Part model, mm, in its own coordinate system. A direction names the side the tool comes from. Give positions to 0.01 mm unless a question says otherwise; leave off trailing zeros. Order: outer loops, then holes, each group sorted by start corner. A loop starts at its lowest first (then second) coordinate and runs counter-clockwise, first axis right, second up. Notation, with made-up numbers: M 9.5,-15.5 L 66.5,-15.5 A16 cw 66.5,-11.5 Z; hole C 34,81.5 d1. An arc over 180 degrees is marked long. Return JSON: item names as keys, results as strings.
Autodesk Inventor part; units mm, degrees
ref_plane "YZ Plane" through (0, 0, 0) normal (1, 0, 0) x (0, 1, 0)
ref_plane "XZ Plane" through (0, 0, 0) normal (0, 1, 0) x (-1, 0, 0)
ref_plane "XY Plane" through (0, 0, 0) normal (0, 0, 1) x (1, 0, 0)
sketch "Boceto1" plane through (0, 0, 0) normal (0, 0, 1) x (1, 0, 0)
  line L0 (0, 0) -> (-1.5875, 0)
  line L1 (-1.4605, 11.9062) -> (0, 11.9062)
  line L2 (0, 11.9062) -> (0, 0)
  line L3 (-1.4605, 11.9062) -> (-1.5875, 11.7793)
  line L4 (-1.1906, 7.5375) -> (-1.1906, 6.7437)
  line L5 (-1.4605, 7.5375) -> (-1.1906, 7.5375)
  line L6 (-1.5875, 7.6645) -> (-1.5875, 11.7793)
  line L7 (-1.5875, 7.6645) -> (-1.4605, 7.5375)
  line L8 (0, 0) -> (-1.905, 0)
  line L9 (-2.3813, 6.7469) -> (-1.1906, 6.7469)
  line L10 (0, 6.7469) -> (0, 0)
  arc A0 (-2.3813, 2.4473) -> (-1.905, 0) centre (-1.905, 1.27) ccw
  line L11 (-2.3813, 0) -> (-2.3813, 0.0927)
  line L12 (-2.3813, 2.4473) -> (-2.3813, 6.7469)
  point P0 (-1.5875, 11.9062)
  point P1 (-1.5875, 7.5375)
  dimension "d0" = 1.5875
  dimension "d1" = 11.9062
  dimension "d2" = 0.127
  dimension "d3" = 0.127
  dimension "d5" = 0.7937
  dimension "d7" = 4.3688
  dimension "d8" = 0.127
  dimension "d9" = 0.127
  dimension "d10" = 2.3813
  dimension "d11" = 6.7469
  dimension "d12" = 2.54
  dimension "d13" = 1.27
  dimension "d14" = 1.905
revolve "Revolución1" add sketch "Boceto1" angle 360 about axis through (0, 11.9062, 0) along (0, -1, 0)
thread "Rosca1"
sketch "Boceto2" plane through (0, 0, 0) normal (0, -1, 0) x (1, 0, 0)
  line L0 (-0.3969, 3.9709) -> (0.3969, 3.9709)
  line L1 (0.3969, 3.9709) -> (0.3969, -4.5285)
  line L2 (0.3969, -4.5285) -> (-0.3969, -4.5285)
  line L3 (-0.3969, -4.5285) -> (-0.3969, 3.9709)
  point P0 (0, 0)
  dimension "d18" = 0.7937
  dimension "d19" = 0.3969
extrude "Extrusión1" cut sketch "Boceto2" against normal blind 0.7937
equation "\"d7\" = d4"
properties part number "Crank Screw" material "Acero inoxidable"
Q1. Band-saw the part on D-D (y = 10.25). Give the cut face in (x, z) (1 decimal), then the cut area to 3 significant figures.
Established:
{"outline": "C 0,0 d3.2", "area": "7.92 mm²"}
Q2. Probe line 1 along Z through (x, y) = (0, 3.25); line 2 along Y through (x, z) = (0.5, 1.25); line 3 along Y through (x, z) = (-1, 1.5). List the from-to ranges inside material, lowest first.
Established:
{"line 1": "z = -2.38 to 2.38", "line 2": "y = 0 to 6.75, 7.54 to 11.91", "line 3": "y = 0 to 6.75"}
Q3. Band-saw the part on C-C (y = 4.75). Give the cut face in (x, z), then the cut area to 3 significant figures.
Established:
{"outline": "C 0,0 d4.76", "area": "17.8 mm²"}
Q4. 3-axis set-ups, long thin cutter, end or side, ignore diameter. For faces 4 (the cylindrical face through (0.34, 9.75, -1.55)), 5 (the flat face through (1, 0, 0)), 6 (the flat face through (1, 6.747, -1)): which of +Z, -Z, +X, -X, +Y, -Y reach the whole face in a straight line?
Established:
{"face 4": "+Y", "face 5": "+Z, -Z, +X, -X, -Y", "face 6": "none"}
Q5. Pin check, flat tips, straight feed: pin 1 (3 mm diameter, centred on x = 2, z = 2.5, fed in from +Y); pin 2 (1 mm diameter, centred on x = -0.5, y = 8, fed in from -Z); pin 3 (1.5 mm diameter, centred on x = 2.5, z = -2, fed in from -Y). Stop position of each tip, or through.
Established:
{"pin 1": "stops at y = 6.75", "pin 2": "stops at z = -1.59", "pin 3": "stops at y = 0.12"}
Q6. Two-plate mould, pull along Y, no slides. Class faces 1 (the cylindrical face through (0.26, 7.14, 1.16)), 2 (the flat face through (-1, 0, 0)), 3 (the cylindrical face through (-1.1, 4.63, -2.11)): +Y half, -Y half, draft (parallel to the pull), parting line (faces both ways), or undercut.
Established:
{"face 1": "undercut", "face 2": "-Y half", "face 3": "draft"}
